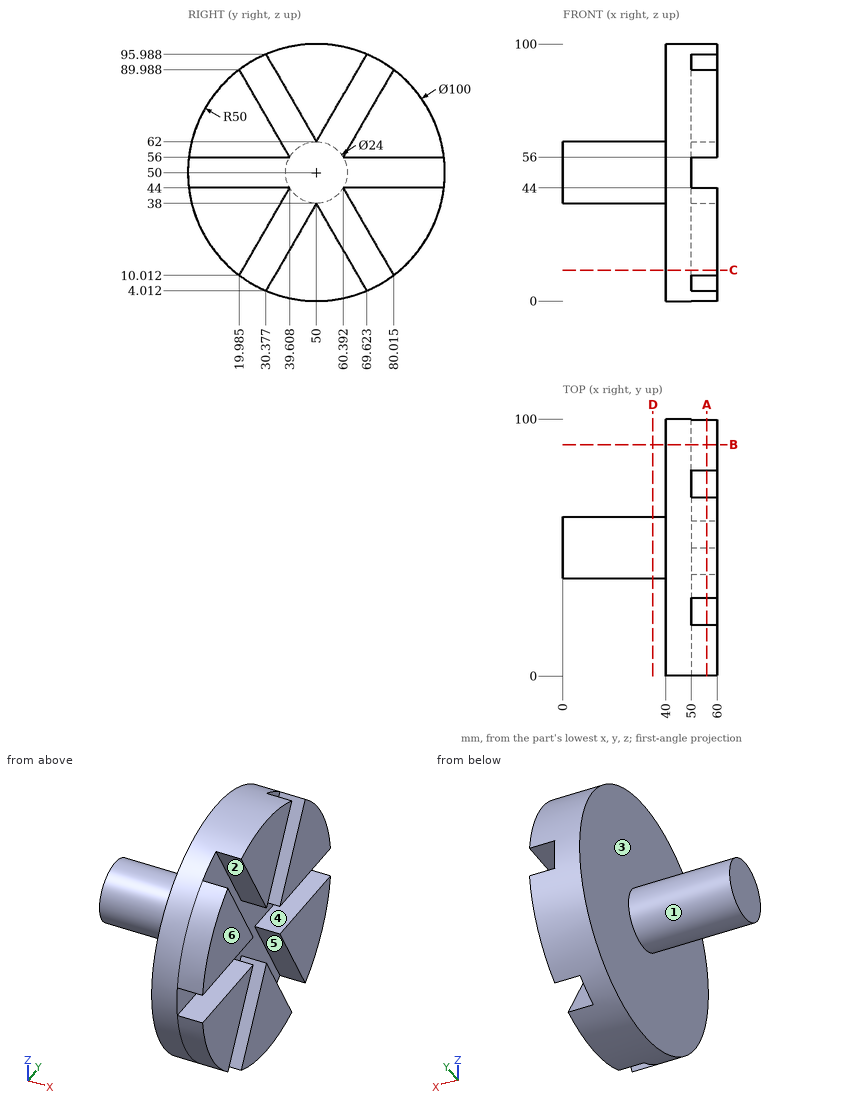
Could you check a few things on this drawing? It's one solid part, dimensions in mm from its lowest x, y, z. A direction names the side the tool comes from. Coordinates: 2 decimals unless noted, no trailing zeros. Loops run counter-clockwise (first coordinate to the right, second up) from the corner with the lowest first, then second, coordinate; pieces in that order, holes last. Notation, with made-up numbers: (66.5, 18.25) - (103.5, 18.25) arc R16 cw to (103.5, 30.25) - close; hole circle Ø1 at (58.5, 0). An arc over 180 degrees is marked (long way). Answer as a JSON object with one key per item and string values. Group by question number.
Item 1: If we section it at D-D (x = 35): List the corners of the cut face in (y, z) for me, plus the area to 3 significant figures.
Item 2: If I drill on L1, parallel to X at y = 30, z = 54; L2, parallel to Z at x = 7, y = 49.5; L3, parallel to X at y = 52.5, z = 50.5, over which ranges is the centre line in solid material (lowest first)? Write a range as from..to.
Item 3: If we mould it in two halves opening along Z, with no side actions, what happens to the marked faces 1, 2 and 3? For each: released by +Z, released by -Z, zero draft, split by the parting line, or undercut.
Item 4: If we section it at C-C (z = 12): List the corners of the cut face in (x, y) for me, plus the area to 3 significant figures.
Item 5: If we section it at B-B (y = 90): List the corners of the cut face in (x, z) for me, plus the area to 3 significant figures.
Item 6: On a 3-axis mill with a long thin cutter (end or side, diameter ignored), from which of +Z, -Z, +X, -X, +Y, -Y can I reach the whole of each face in a straight line? I mean the marked faces 4, 5 and 6. Say none if no direction works.
Item 7: For pin 1 (1.5 mm diameter, centred on x = 40.5, y = 70.5, fed in from -Z) (1 decimal); pin 2 (1.5 mm diameter, centred on x = 42.5, y = 48, fed in from -Z); pin 3 (3 mm diameter, centred on x = 56, y = 88.5, fed in from +Z), each with a flat end and sliding along its axis, tell me the tip position at first contact or that it passes through.
Item 8: If we section it at A-A (x = 56): List the corners of the cut face in (y, z) for me (1 decimal), plus the area to 3 significant figures.
Returned:
{
 "1": {"outline": "circle Ø24 at (50, 50)", "area": "452 mm²"},
 "2": {"L1": "x = 40..50", "L2": "z = 38.01..61.99", "L3": "x = 0..50"},
 "3": {"face 1": "split by the parting line", "face 2": "undercut", "face 3": "zero draft"},
 "4": {"outline": "(40, 17.5) - (60, 17.5) - (60, 21.13) - (50, 21.13) - (50, 34.99) - (60, 34.99) - (60, 65.01) - (50, 65.01) - (50, 78.87) - (60, 78.87) - (60, 82.5) - (40, 82.5) - close", "area": "1,020 mm²"},
 "5": {"outline": "(40, 20) - (60, 20) - (60, 44) - (50, 44) - (50, 56) - (60, 56) - (60, 80) - (40, 80) - close", "area": "1,080 mm²"},
 "6": {"face 4": "+X, +Y, -Y", "face 5": "+X", "face 6": "+Z, -Z, +X, +Y, -Y"},
 "7": {"pin 1": "stops at z = 4.1", "pin 2": "stops at z = 0.02", "pin 3": "stops at z = 83.63"},
 "8": {"outline": "(0.4, 44) arc R50 ccw to (20, 10) - (39.6, 44) - close; (0.4, 56) - (39.6, 56) - (20, 90) arc R50 ccw to start; (30.4, 4) arc R50 ccw to (69.6, 4) - (50, 38) - close; (30.4, 96) - (50, 62) - (69.6, 96) arc R50 ccw to start; (60.4, 44) - (80, 10) arc R50 ccw to (99.6, 44) - close; (60.4, 56) - (99.6, 56) arc R50 ccw to (80, 90) - close", "area": "4,640 mm²"}
}
